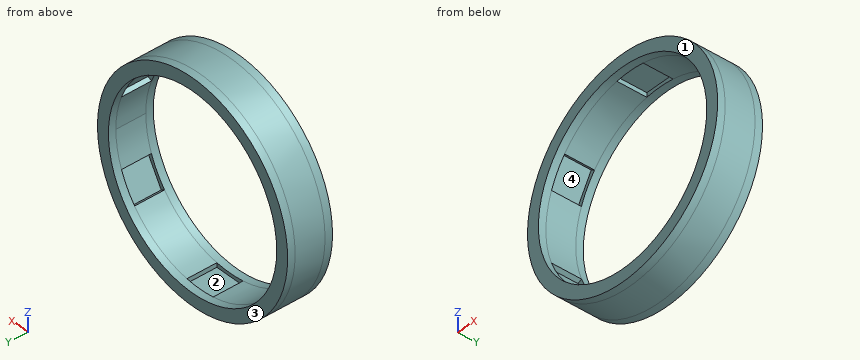
from build123d import *

# Parameters (mm, degrees)
F0_R     = 43.5
F1_DEPTH = 6
F2_R     = 43.5
F2_R_2   = 38.5
F3_DEPTH = 3
F4_R     = 43.5
F4_R_2   = 38.5
F5_DEPTH = 3


with BuildPart() as f1:
    # F0 (on Front) → F1 (new body, symmetric)
    with BuildSketch(Plane.XZ):
        Circle(F0_R)
        with BuildLine():
            Line((-6, 38.029594), (-6, 39.784067))
            Line((-6, 39.784067), (6, 39.784067))
            Line((6, 39.784067), (6, 38.029594))
            ThreePointArc((6, 38.029594), (19.25, 33.341978), (29.934594, 24.210949))
            Line((29.934594, 24.210949), (31.454013, 25.088186))
            Line((31.454013, 25.088186), (37.454013, 14.695881))
            Line((37.454013, 14.695881), (35.934594, 13.818644))
            ThreePointArc((35.934594, 13.818644), (37.853216, 7.027379), (38.5, 0))
            ThreePointArc((38.5, 0), (37.853216, -7.027379), (35.934594, -13.818644))
            Line((35.934594, -13.818644), (37.454013, -14.695881))
            Line((37.454013, -14.695881), (31.454013, -25.088186))
            Line((31.454013, -25.088186), (29.934594, -24.210949))
            ThreePointArc((29.934594, -24.210949), (19.25, -33.341978), (6, -38.029594))
            Line((6, -38.029594), (6, -39.784067))
            Line((6, -39.784067), (-6, -39.784067))
            Line((-6, -39.784067), (-6, -38.029594))
            ThreePointArc((-6, -38.029594), (-19.25, -33.341978), (-29.934594, -24.210949))
            Line((-29.934594, -24.210949), (-31.454013, -25.088186))
            Line((-31.454013, -25.088186), (-37.454013, -14.695881))
            Line((-37.454013, -14.695881), (-35.934594, -13.818644))
            ThreePointArc((-35.934594, -13.818644), (-38.5, 0), (-35.934594, 13.818644))
            Line((-35.934594, 13.818644), (-37.454013, 14.695881))
            Line((-37.454013, 14.695881), (-31.454013, 25.088186))
            Line((-31.454013, 25.088186), (-29.934594, 24.210949))
            ThreePointArc((-29.934594, 24.210949), (-19.25, 33.341978), (-6, 38.029594))
        make_face(mode=Mode.SUBTRACT)
    extrude(amount=F1_DEPTH, both=True)

    # F2 (on face) → F3 (join)
    with BuildSketch(Plane(origin=(0, 6, 0), x_dir=(-1, 0, 0), z_dir=(0, 1, 0))):
        Circle(F2_R)
        Circle(F2_R_2, mode=Mode.SUBTRACT)
    extrude(amount=F3_DEPTH)

    # F4 (on face) → F5 (join)
    with BuildSketch(Plane.XZ.offset(6)):
        Circle(F4_R)
        Circle(F4_R_2, mode=Mode.SUBTRACT)
    extrude(amount=F5_DEPTH)


solid = f1.part
Can you work these out from the model? Positions are in its coordinate system, mm. Face numbers are marked on the shaded views. A direction names the side the tool comes from. Round coordinates to 2 decimals unless told otherwise and drop trailing zeros. Loops run counter-clockwise (first coordinate to the right, second up) from the corner with the lowest first, then second, coordinate; pieces in that order, holes last. Notation, with made-up numbers: (5.25, -2.5) - (23.25, -2.5) arc R25 ccw to (23.25, 12.5) - close; hole circle Ø10 at (7, -28.75). An arc over 180 degrees is marked (long way). Answer in a Markdown table with one row per item. Add a question column.
Q1. Which directions (+Z, -Z, +X, -X, +Y, -Y) give clear straight access to the entire face, cutting with the end or side of a thin tool? Please do the marked faces 1 and 2.
Q2. I want a section at C-C on y = -3.75. List the corners of the cut face in (x, z) for me.
Q3. For pin 1 Ø8 at (y, z) = (-5.5, 13) entering from -X; pin 2 Ø1.4 at (y, z) = (2, -38.5) entering from -X; pin 3 Ø6 at (x, y) = (-0.5, 1.5) entering from -Z, each with a flat end and sliding along its axis, tell me the tip position at first contact or that it passes through.
Q4. I want a section at A-A on x = 0. List the corners of the cut face in (y, z) for me, and give its area (3 significant figures).
Q5. I need wall thicknesses on L1, parallel to X at y = 8, z = 0; L2, parallel to Z at x = -0.5, y = 3. Which ranges of each line are inside material? Lowest first, please.
Q6. I want a section at D-D on x = 17. List the corners of the cut face in (y, z) for me.
Q7. I want a section at B-B on z = 34. List the corners of the cut face in (x, y) for me, and give its area (3 significant figures).
Q8. We'd pull the mould along Z, two halves only. Please class the marked faces 3 and 4: pulls with the +Z half, pulls with the -Z half, needs draft (parallel to the pull), parting line crosses it, or undercut.
A:
| question | item | result |
|---|---|---|
| 1 | face 1 | +Z, -Z, +X, -X, -Y |
| 1 | face 2 | none |
| 2 | outline | circle Ø87 at (0, 0); hole (-37.45, -14.7) - (-31.45, -25.09) - (-29.93, -24.21) arc R38.5 ccw to (-6, -38.03) - (-6, -39.78) - (6, -39.78) - (6, -38.03) arc R38.5 ccw to (29.93, -24.21) - (31.45, -25.09) - (37.45, -14.7) - (35.93, -13.82) arc R38.5 ccw to (38.5, 0) arc R38.5 ccw to (35.93, 13.82) - (37.45, 14.7) - (31.45, 25.09) - (29.93, 24.21) arc R38.5 ccw to (6, 38.03) - (6, 39.78) - (-6, 39.78) - (-6, 38.03) arc R38.5 ccw to (-29.93, 24.21) - (-31.45, 25.09) - (-37.45, 14.7) - (-35.93, 13.82) arc R38.5 ccw to (-35.93, -13.82) - close |
| 3 | pin 1 | x = -42.56 |
| 3 | pin 2 | x = -21.53 |
| 3 | pin 3 | z = -43.5 |
| 4 | outline | (-9, -43.5) - (9, -43.5) - (9, -38.5) - (6, -38.5) - (6, -39.78) - (-6, -39.78) - (-6, -38.5) - (-9, -38.5) - close; (-9, 38.5) - (-6, 38.5) - (-6, 39.78) - (6, 39.78) - (6, 38.5) - (9, 38.5) - (9, 43.5) - (-9, 43.5) - close |
| 4 | area | 149 mm^2 |
| 5 | L1 | -43.5 to -38.5, 38.5 to 43.5 |
| 5 | L2 | -43.5 to -39.78, 39.78 to 43.5 |
| 6 | outline | (-9, -40.04) - (9, -40.04) - (9, -34.54) - (-9, -34.54) - close; (-9, 34.54) - (9, 34.54) - (9, 40.04) - (-9, 40.04) - close |
| 7 | outline | (-27.13, -9) - (-18.06, -9) - (-18.06, 9) - (-27.13, 9) - close; (18.06, -9) - (27.13, -9) - (27.13, 9) - (18.06, 9) - close |
| 7 | area | 327 mm^2 |
| 8 | face 3 | needs draft |
| 8 | face 4 | undercut |
